Job drawing, mm, ordinate dimensions from the low corner. One solid piece. A direction names the side the tool comes from. Round coordinates to 2 decimals unless told otherwise and drop trailing zeros. Loops run counter-clockwise (first coordinate to the right, second up) from the corner with the lowest first, then second, coordinate; pieces in that order, holes last. Notation, with made-up numbers: (81, -26) - (111, -26) arc R27 ccw to (111, -4) - close; hole circle Ø9 at (54.5, 24.25). An arc over 180 degrees is marked (long way). One line per question, with ' | ' between items. Start each with the question number.
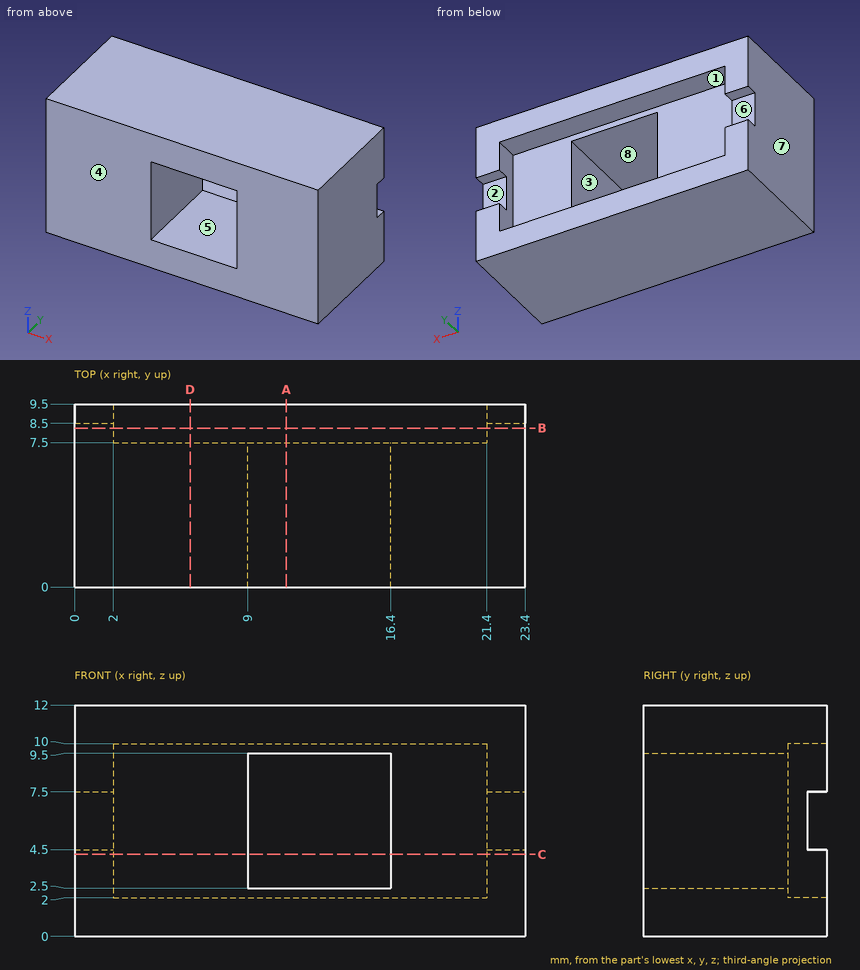
1) Tool access for the marked faces 1, 2, 3 and 4: list every direction of +Z, -Z, +X, -X, +Y, -Y with a clear straight run to the whole face (end or side of a thin tool).
2) Wall check: line 1 (X direction, y = 1.75, z = 3.5); line 2 (X direction, y = 8, z = 7); line 3 (Z direction, x = 8.75, y = 8.75). Give the ranges that are in metal, low to high. Write a range as [from, to].
3) Saw through at B-B on y = 8.25. Write the cut outline in (x, z), and give its area (3 significant figures).
4) Saw through at C-C on z = 4.25. Write the cut outline in (x, y), and give its area (3 significant figures).
5) Two-plate mould, pull along X, no slides. Class the marked faces 5, 6, 7 and 8: +X half, -X half, draft (parallel to the pull), parting line (faces both ways), or undercut.
6) Saw through at D-D on x = 6. Write the cut outline in (y, z), and give its area (3 significant figures).
7) Saw through at A-A on x = 11. Write the cut outline in (y, z).
8) Drop a flat-ended pin along its axis: pin 1 (1.6 mm diameter, centred on x = 1.5, z = 5.5, fed in from +Y). Give the stop position or say it passes through.
Answer key:
1) face 1: +Y | face 2: +X, -X, +Y | face 3: +Y, -Y | face 4: +Z, -Z, +X, -X, -Y
2) line 1: [0, 9], [16.4, 23.4] | line 2: [0, 2], [21.4, 23.4] | line 3: [0, 2], [10, 12]
3) outline: (0, 0) - (23.4, 0) - (23.4, 12) - (0, 12) - close; hole (2, 2) - (21.4, 2) - (21.4, 10) - (2, 10) - close | area: 126 mm²
4) outline: (0, 0) - (9, 0) - (9, 7.5) - (2, 7.5) - (2, 9.5) - (0, 9.5) - close; (16.4, 0) - (23.4, 0) - (23.4, 9.5) - (21.4, 9.5) - (21.4, 7.5) - (16.4, 7.5) - close | area: 128 mm²
5) face 5: undercut | face 6: draft | face 7: -X half | face 8: undercut
6) outline: (0, 0) - (9.5, 0) - (9.5, 2) - (7.5, 2) - (7.5, 10) - (9.5, 10) - (9.5, 12) - (0, 12) - close | area: 98.0 mm²
7) outline: (0, 0) - (9.5, 0) - (9.5, 2) - (7.5, 2) - (7.5, 2.5) - (0, 2.5) - close; (0, 9.5) - (7.5, 9.5) - (7.5, 10) - (9.5, 10) - (9.5, 12) - (0, 12) - close
8) pin 1: y = 8.5
